```python
from build123d import *

# Parameters (mm, degrees)
SKETCH1_W           = 188.976
SKETCH1_H           = 10.922
BOSS_EXTRUDE1_DEPTH = 3.175
FILLET1_R           = 5.588
SKETCH2_R           = 1.4605
CUT_EXTRUDE1_DEPTH  = 95.697479006


with BuildPart() as part:
    # Sketch1 → Boss-Extrude1 (new body)
    with BuildSketch(Plane.XY):
        Rectangle(SKETCH1_W, SKETCH1_H)
    extrude(amount=BOSS_EXTRUDE1_DEPTH)

    # Fillet1
    # the kernel refuses this fillet: 5.588 mm, written as the material it takes off along each edge
    with BuildSketch(Plane(origin=(-94.488, -5.461, -13.97), x_dir=(1, 0, 0), z_dir=(0, 0, 1))) as fillet1_piece_1:
        with BuildLine():
            CenterArc((FILLET1_R, FILLET1_R), FILLET1_R, 180, 90)
            Line((0, FILLET1_R), (0, 0))
            Line((0, 0), (FILLET1_R, 0))
        make_face()
    extrude(amount=31.115, mode=Mode.SUBTRACT)
    with BuildSketch(Plane(origin=(-94.488, 5.461, -13.97), x_dir=(1, 0, 0), z_dir=(0, 0, 1)), Plane(origin=(94.488, -5.461, -13.97), x_dir=(-1, 0, 0), z_dir=(0, 0, 1)), Plane(origin=(94.488, 5.461, -13.97), x_dir=(0, -1, 0), z_dir=(0, 0, 1))) as fillet1_piece_2:
        with BuildLine():
            CenterArc((FILLET1_R, -FILLET1_R), FILLET1_R, 90, 90)
            Line((0, -FILLET1_R), (0, 0))
            Line((0, 0), (FILLET1_R, 0))
        make_face()
    extrude(amount=31.115, mode=Mode.SUBTRACT)

    # Sketch2 → Cut-Extrude1 (cut, through all)
    with BuildSketch(Plane.XY.offset(3.175)):
        with Locations((-88.9, -0.127)):
            Circle(SKETCH2_R)
        with Locations((88.9, -0.127)):
            Circle(SKETCH2_R)
    extrude(amount=-CUT_EXTRUDE1_DEPTH, mode=Mode.SUBTRACT)


solid = part.part
```
Read the model definition and answer for the solid it produces. Units are mm, in the model's axes. Round coordinates to 2 decimals unless told otherwise and drop trailing zeros. Write each loop counter-clockwise with the first axis right and the second up, starting at its lowest first coordinate (ties: lowest second). Pieces come first, ordered by that corner, then holes. Notation, with made-up numbers: (82.5, -38.75) - (123.5, -38.75) arc R16 cw to (123.5, -11.75) - close; hole circle Ø2 at (-20.5, -32.75). An arc over 180 degrees is marked (long way). One line per item, written item: value.
Q1. Straight lines are drawn through the part: line 1 (X direction, y = 0.5, z = 0.5); line 2 (Y direction, x = -88.9, z = 1.75); line 3 (X direction, y = -1, z = 1.4). For each, find the intervals that lie inside material, in ascending order. Write a range as from..to.
The answers:
line 1: x = -94.45..-90.22, -87.58..87.58, 90.22..94.45
line 2: y = -5.46..-1.59, 1.33..5.46
line 3: x = -94.37..-90.07, -87.73..87.73, 90.07..94.37
Q2. Find section A-A (z = 2.45). Determine the outline of the cut face in (x, y).
The answers:
outline: (-94.49, 0) arc R5.59 ccw to (-88.9, -5.46) - (88.9, -5.46) arc R5.59 ccw to (94.49, 0) arc R5.59 ccw to (88.9, 5.46) - (-88.9, 5.46) arc R5.59 ccw to start; hole circle Ø2.92 at (-88.9, -0.13); hole circle Ø2.92 at (88.9, -0.13)
Q3. For a pull along X with two mould halves and no side action, classify faces 1 (the flat face through (-1, 5.461, 2)), 2 (the cylindrical face through (-90.36, -0.06, 1.61)), 3 (the cylindrical face through (92.849, 3.826, 1.565)) as pulls with the +X half, pulls with the -X half, needs draft (parallel to the pull), parting line crosses it, or undercut.
The answers:
face 1: needs draft
face 2: undercut
face 3: pulls with the +X half
Q4. This flat-tipped pin is pushed along its axis until it touches: P1, Ø2.5, axis at x = 88.9, y = -0.127, coming from the -Z side. Where does it stop, or does it pass through?
The answers:
P1: passes through
